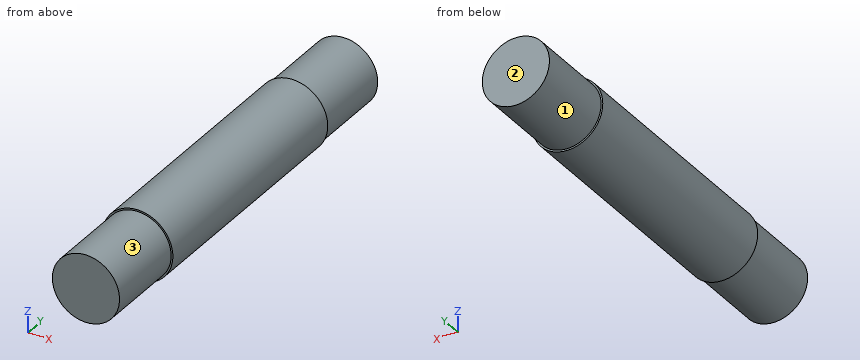
Autodesk Inventor part; units mm, degrees
ref_plane "YZ Plane" through (0, 0, 0) normal (1, 0, 0) x (0, 1, 0)
ref_plane "XZ Plane" through (0, 0, 0) normal (0, 1, 0) x (-1, 0, 0)
ref_plane "XY Plane" through (0, 0, 0) normal (0, 0, 1) x (1, 0, 0)
sketch "Sketch1" plane through (0, 0, 0) normal (0, 0, 1) x (1, 0, 0)
  line L0 (0, 0) -> (-2, 0)
  line L1 (-2, 25) -> (0, 25)
  line L2 (0, 25) -> (0, 0)
  line L3 (-2, 25) -> (-2, 20)
  line L4 (-2, 20) -> (-2.1, 20)
  line L5 (-2.1, 20) -> (-2.1, 5)
  line L6 (-2.1, 5) -> (-2, 5)
  line L7 (-2, 5) -> (-2, 0)
  dimension "d0" = 2
  dimension "d7" = 2.1
  dimension "d12" = 5
  dimension "d13" = 5
  dimension "d14" = 25
revolve "Revolution1" add sketch "Sketch1" angle 360 about axis through (0, 25, 0) along (0, -1, 0)
thread "Thread2"
properties part number "FrameSupport-Link" material "Copper"
Verification items for the finished model (mm, model axes). Face numbers are marked on the shaded views. A direction names the side the tool comes from. Coordinates: 2 decimals unless noted, no trailing zeros. Loops run counter-clockwise (first coordinate to the right, second up) from the corner with the lowest first, then second, coordinate; pieces in that order, holes last. Notation, with made-up numbers: (-6.75, -21.75) -> (37.25, -21.75) arc R29 cw to (37.25, 3.25) -> close; hole circle Ø1 at (76.25, 45.25). An arc over 180 degrees is marked (long way). Answer as a JSON object with one key per item and string values. Group by question number.
Item 1: Tool access check on the marked faces 1, 2 and 3. Record the directions out of +Z, -Z, +X, -X, +Y, -Y that give a thin tool (end or side, any length) a straight path to the whole face; none if there is none.
Item 2: Sectioned sample at D-D on y = 3.75. Record the boundary of the cut face in (x, z), plus the area to 3 significant figures.
Item 3: Scan lines: probe 1 along X at (y, z) = (19.5, -1.7); probe 2 along Z at (x, y) = (0.25, 17.75); probe 3 along X at (y, z) = (11.25, -1.4). Record each from-to range of solid material in increasing order.
Item 4: Sectioned sample at A-A on x = 0. Record the boundary of the cut face in (y, z), plus the area to 3 significant figures.
Item 5: Depth check by flat-ended pin: pin 1 (2 mm diameter, centred on y = 3.5, z = 1.5, fed in from -X). Enter the tip coordinate at first touch or a pass-through.
Item 6: Sectioned sample at C-C on y = 6.75. Record the boundary of the cut face in (x, z).
Item 7: Sectioned sample at B-B on z = 0. Record the boundary of the cut face in (x, y), plus the area to 3 significant figures.
Evaluation:
{
 "1": {"face 1": "+Y", "face 2": "+Z, -Z, +X, -X, +Y", "face 3": "-Y"},
 "2": {"outline": "circle Ø4 at (0, 0)", "area": "12.6 mm²"},
 "3": {"probe 1": "x = -1.23 to 1.23", "probe 2": "z = -2.09 to 2.09", "probe 3": "x = -1.57 to 1.57"},
 "4": {"outline": "(0, -2) -> (5, -2) -> (5, -2.1) -> (20, -2.1) -> (20, -2) -> (25, -2) -> (25, 2) -> (20, 2) -> (20, 2.1) -> (5, 2.1) -> (5, 2) -> (0, 2) -> close", "area": "103 mm²"},
 "5": {"pin 1": "stops at x = -1.94"},
 "6": {"outline": "circle Ø4.2 at (0, 0)"},
 "7": {"outline": "(-2.1, 5) -> (-2, 5) -> (-2, 0) -> (2, 0) -> (2, 5) -> (2.1, 5) -> (2.1, 20) -> (2, 20) -> (2, 25) -> (-2, 25) -> (-2, 20) -> (-2.1, 20) -> close", "area": "103 mm²"}
}
